from build123d import *

# Parameters (mm, degrees)
SKETCH1_W           = 165.1
SKETCH1_H           = 90
BOSS_EXTRUDE1_DEPTH = 5
SKETCH2_R           = 1.45
CUT_EXTRUDE1_DEPTH  = 7
SKETCH4_W           = 165.1
SKETCH4_H           = 90
BOSS_EXTRUDE2_DEPTH = 3.5
CHAMFER1_SIZE       = 3.5
CHAMFER1_SIZE2      = 4.171137574
SKETCH5_W           = 100.2
SKETCH5_H           = 79.2
CUT_EXTRUDE3_DEPTH  = 6.5
SKETCH8_R           = 1.45
CUT_EXTRUDE5_DEPTH  = 3
SKETCH10_W          = 165.1
SKETCH10_H          = 8.5
BOSS_EXTRUDE4_DEPTH = 17
FILLET1_R           = 3


with BuildPart() as part:
    # Sketch1 → Boss-Extrude1 (new body)
    with BuildSketch(Plane.XY):
        with Locations((0, -35.801949153)):
            Rectangle(SKETCH1_W, SKETCH1_H)
    extrude(amount=BOSS_EXTRUDE1_DEPTH)

    # Sketch2 → Cut-Extrude1 (cut)
    with BuildSketch(Plane(origin=(0, 9.198050847, 0), x_dir=(1, 0, 0), z_dir=(0, 1, 0))):
        with Locations(Location((-80.05, -2.5, 0), (0, 0, 270))):
            Circle(SKETCH2_R)
        with Locations(Location((80.05, -2.5, 0), (0, 0, 270))):
            Circle(SKETCH2_R)
    extrude(amount=-CUT_EXTRUDE1_DEPTH, mode=Mode.SUBTRACT)

    # Sketch4 → Boss-Extrude2 (add)
    with BuildSketch(Plane(origin=(0, 0, 0), x_dir=(-1, 0, 0), z_dir=(0, 0, -1))):
        with Locations((0, -35.801949153)):
            Rectangle(SKETCH4_W, SKETCH4_H)
    extrude(amount=BOSS_EXTRUDE2_DEPTH)

    # Chamfer1
    chamfer1_edges = [part.edges().sort_by_distance(p)[0] for p in [
        (0, 9.198050847, -3.5),
    ]]
    chamfer1_side = [part.faces().sort_by_distance(p)[0] for p in [
        (0, 9.198050847, 0.733369875),
    ]]
    chamfer(chamfer1_edges, length=CHAMFER1_SIZE, length2=CHAMFER1_SIZE2, reference=chamfer1_side[0])

    # Sketch5 → Cut-Extrude3 (cut)
    with BuildSketch(Plane(origin=(0, 0, -3.5), x_dir=(-1, 0, 0), z_dir=(0, 0, -1))):
        with Locations((0, -35.801949153)):
            Rectangle(SKETCH5_W, SKETCH5_H)
    extrude(amount=-CUT_EXTRUDE3_DEPTH, mode=Mode.SUBTRACT)

    # Sketch8 → Cut-Extrude5 (cut)
    with BuildSketch(Plane(origin=(82.55, 0, 0), x_dir=(0, 0, -1), z_dir=(1, 0, 0))):
        with Locations((0.5, -66.551949153)):
            Circle(SKETCH8_R)
    cut_extrude5 = extrude(amount=-CUT_EXTRUDE5_DEPTH, mode=Mode.SUBTRACT)

    # Mirror2: Cut-Extrude5 across plane
    add(cut_extrude5.mirror(Plane(origin=(0, 0, 0), x_dir=(0, 0, 1), z_dir=(1, 0, 0))), mode=Mode.SUBTRACT)

    # Sketch10 → Boss-Extrude4 (add)
    with BuildSketch(Plane.XZ.offset(80.801949153)):
        with Locations((0, 0.75)):
            Rectangle(SKETCH10_W, SKETCH10_H)
    extrude(amount=BOSS_EXTRUDE4_DEPTH)

    # Fillet1
    fillet1_edges = [part.edges().sort_by_distance(p)[0] for p in [
        (-82.55, -97.801949153, 0.75),
        (82.55, -97.801949153, 0.75),
    ]]
    fillet(fillet1_edges, radius=FILLET1_R)


solid = part.part
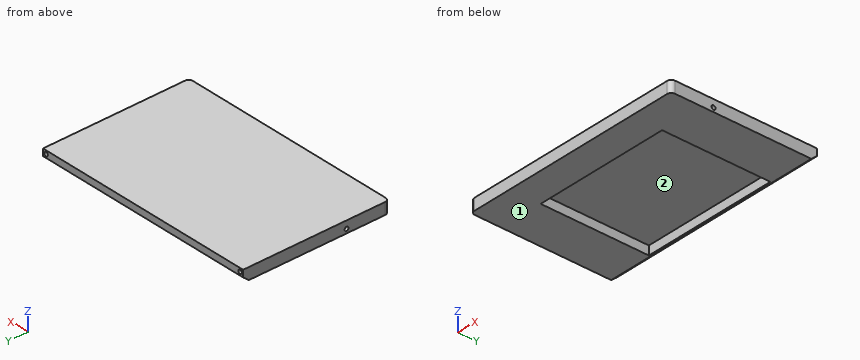
CAD build for the part. Positions are in the model's coordinates, mm. Face numbers are marked on the shaded views. Round coordinates to 2 decimals unless told otherwise and drop trailing zeros. Loops run counter-clockwise (first coordinate to the right, second up) from the corner with the lowest first, then second, coordinate; pieces in that order, holes last.
(1) Cut at B-B (y = -1). Give the cut face in (x, z).
(2) Cut at A-A (x = 19.5). Give the cut face in (y, z).
(3) Two-plate mould, pull along X, no slides. Class the marked faces 1 and 2: +X half, -X half, draft (parallel to the pull), parting line (faces both ways), or undercut.
(4) Drop flat-ended pins along their axis: pin 1 (3.5 mm diameter, centred on y = -66.55, z = -0.5, fed in from +X); pin 2 (0.9 mm diameter, centred on y = -66, z = -0.5, fed in from +X); pin 3 (4 mm diameter, centred on x = 44.5, y = -48.5, fed in from -Z); pin 4 (1.4 mm diameter, centred on y = -66, z = -0.5, fed in from -X). Give the stop position or say it passes through.
(5) Wall check: line 1 along X through (y, z) = (6.5, 2.5); line 2 along X through (y, z) = (-22, -0.5); line 3 along Y through (x, z) = (-50, 1). Give the ranges that are in metal, low to high.
Findings below:
1. outline: (-82.55, -3.5) - (-50.1, -3.5) - (-50.1, 3) - (50.1, 3) - (50.1, -3.5) - (82.55, -3.5) - (82.55, 5) - (-82.55, 5) - close
2. outline: (-97.8, -3.5) - (-75.4, -3.5) - (-75.4, 3) - (3.8, 3) - (3.8, -3.5) - (5.03, -3.5) - (9.2, 0) - (9.2, 5) - (-97.8, 5) - close
3. face 1: draft
3. face 2: undercut
4. pin 1: stops at x = 82.55
4. pin 2: stops at x = 79.55
4. pin 3: stops at z = 3
4. pin 4: stops at x = -79.55
5. line 1: x = -82.55 to -81.5, -78.6 to 78.6, 81.5 to 82.55
5. line 2: x = -82.55 to -50.1, 50.1 to 82.55
5. line 3: y = -97.8 to -75.4, 3.8 to 9.2
